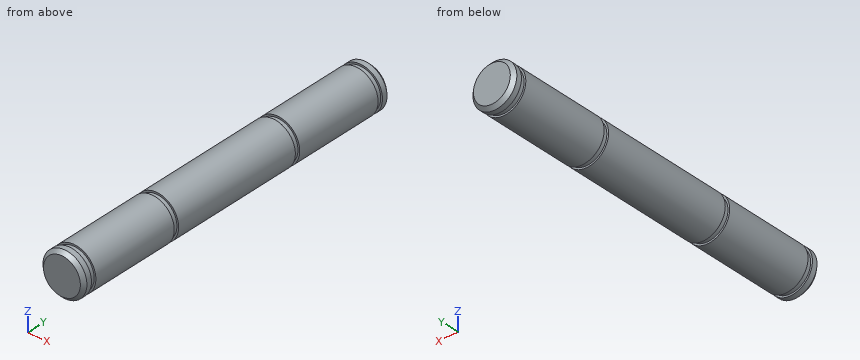
from build123d import *

# Parameters (mm, degrees)
CHAMFER1_SIZE = 0.508


with BuildPart() as part:
    # Sketch1 → Revolve1 (revolve)
    with BuildSketch(Plane.XY):
        Polygon((-3.175, 23.5585), (-3.175, 10.4775), (-2.921, 10.4775), (-2.921, 9.7409), (-3.175, 9.7409), (-3.175, -9.7409), (-2.921, -9.7409), (-2.921, -10.4775), (-3.175, -10.4775), (-3.175, -23.5585), (-2.921, -23.5585), (-2.921, -24.2951), (-3.175, -24.2951), (-3.175, -25.5651), (0, -25.5651), (0, 25.5651), (-3.175, 25.5651), (-3.175, 24.2951), (-2.921, 24.2951), (-2.921, 23.5585), align=None)
    revolve(axis=Axis((0, 25.5651, 0), (0, -1, 0)))

    # Chamfer1
    chamfer1_edges = [part.edges().sort_by_distance(p)[0] for p in [
        (3.175, 25.5651, 0),
        (3.175, -25.5651, 0),
    ]]
    chamfer(chamfer1_edges, length=CHAMFER1_SIZE)


solid = part.part
Check sheet for the modelled part. Datum: model origin and axes. Units: mm. Give positions to 0.01 mm unless a question says otherwise; leave off trailing zeros. Write each loop counter-clockwise with the first axis right and the second up, starting at its lowest first coordinate (ties: lowest second). Pieces come first, ordered by that corner, then holes. Notation, with made-up numbers: M 47.5,55.25 L 80.5,55.25 A21 ccw 80.5,62.25 Z; hole C 88.25,47 d4. An arc over 180 degrees is marked long. Use one line per item in the form item = value.
(1) Section check A-A on y = 14. Record the boundary of the cut face in (x, z) (3 decimals).
Answer block:
outline = C 0,0 d6.35
(2) Depth check by flat-ended pin: P1, Ø1, axis at x = 1.5, y = 6.5, coming from the +Z side; P2, Ø1, axis at y = -4.5, z = -2, coming from the +X side. Enter the tip coordinate at first touch or a pass-through.
Answer block:
P1 = 3.01
P2 = 2.8
(3) Material ranges on line 1 along X through (y, z) = (-17.5, 0.25); line 2 along Z through (x, y) = (-1.25, 3), recorded low to high.
Answer block:
line_1 = -3.17 to 3.17
line_2 = -2.92 to 2.92
